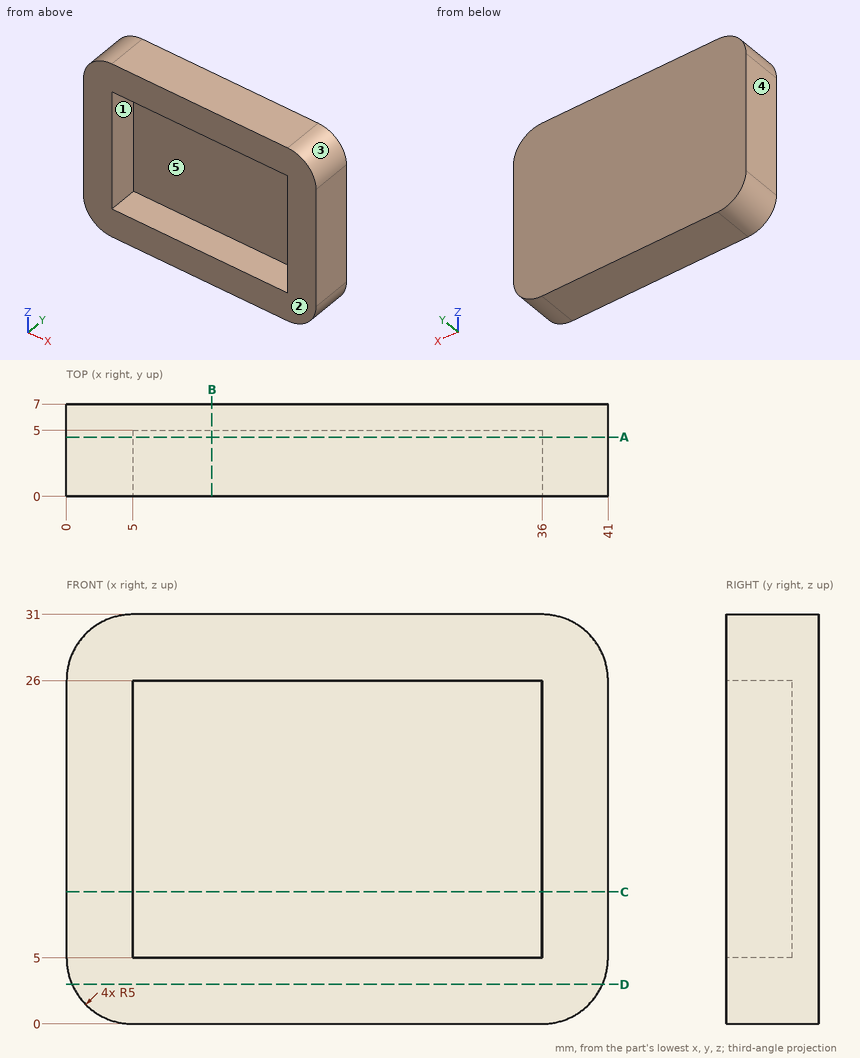
Geometry check sheet. Reference: drawing and pictorial views, mm from the part's lowest x, y, z. A direction names the side the tool comes from. Give positions to 0.01 mm unless a question says otherwise; leave off trailing zeros. Order: outer loops, then holes, each group sorted by start corner. A loop starts at its lowest first (then second) coordinate and runs counter-clockwise, first axis right, second up. Notation, with made-up numbers: M 72.5,64.5 L 120.5,64.5 A29 ccw 120.5,103.5 Z; hole C 6,50.5 d8. An arc over 180 degrees is marked long. Return JSON: item names as keys, results as strings. Group by question number.
1) Section check A-A on y = 4.5. Record the cut outline in (x, z).
2) Mould release check, pull along X, two halves, no side actions. Record for the marked faces 1, 2 and 3: pulls with the +X half, pulls with the -X half, needs draft (parallel to the pull), parting line crosses it, or undercut.
3) Scan lines: line 1 (Z direction, x = 8, y = 3.5); line 2 (X direction, y = 4, z = 17.5); line 3 (Y direction, x = 7, z = 21). Record each from-to range of solid material in increasing order.
4) Section check D-D on z = 3. Record the cut outline in (x, y), and give its area (3 significant figures).
5) Section check C-C on z = 10. Record the cut outline in (x, y), and give its area (3 significant figures).
6) Go/stop test with flat-tipped pins: pin 1 Ø1 at (y, z) = (2, 6.5) entering from -X; pin 2 Ø1 at (x, z) = (25.5, 15.5) entering from -Y. Record where each tip stops, or that it passes through.
7) Access from +Z, -Z, +X, -X, +Y, -Y to the whole of each face (thin tool, end or side, straight path). Record for the marked faces 4 and 5.
8) Section check B-B on x = 11. Record the cut outline in (y, z).
Answer block:
{
 "1": {"outline": "M 0,5 A5 ccw 5,0 L 36,0 A5 ccw 41,5 L 41,26 A5 ccw 36,31 L 5,31 A5 ccw 0,26 Z; hole M 5,5 L 36,5 L 36,26 L 5,26 Z"},
 "2": {"face 1": "undercut", "face 2": "needs draft", "face 3": "pulls with the +X half"},
 "3": {"line 1": "z = 0 to 5, 26 to 31", "line 2": "x = 0 to 5, 36 to 41", "line 3": "y = 5 to 7"},
 "4": {"outline": "M 0.42,0 L 40.58,0 L 40.58,7 L 0.42,7 Z", "area": "281 mm^2"},
 "5": {"outline": "M 0,0 L 5,0 L 5,5 L 36,5 L 36,0 L 41,0 L 41,7 L 0,7 Z", "area": "132 mm^2"},
 "6": {"pin 1": "stops at x = 0", "pin 2": "stops at y = 5"},
 "7": {"face 4": "+Z, -Z, -X, +Y, -Y", "face 5": "-Y"},
 "8": {"outline": "M 0,0 L 7,0 L 7,31 L 0,31 L 0,26 L 5,26 L 5,5 L 0,5 Z"}
}
